Could you check a few things on this model? Use its own coordinates, in mm. Face numbers are marked on the shaded views. Coordinates: 2 decimals unless noted, no trailing zeros. Loops run counter-clockwise (first coordinate to the right, second up) from the corner with the lowest first, then second, coordinate; pieces in that order, holes last. Notation, with made-up numbers: (37.5, 73) - (62.5, 73) arc R10 cw to (62.5, 78) - close; hole circle Ø2 at (-3.5, 8.25). An arc over 180 degrees is marked (long way). Use CSV: the item, a comma, the result in double quotes.
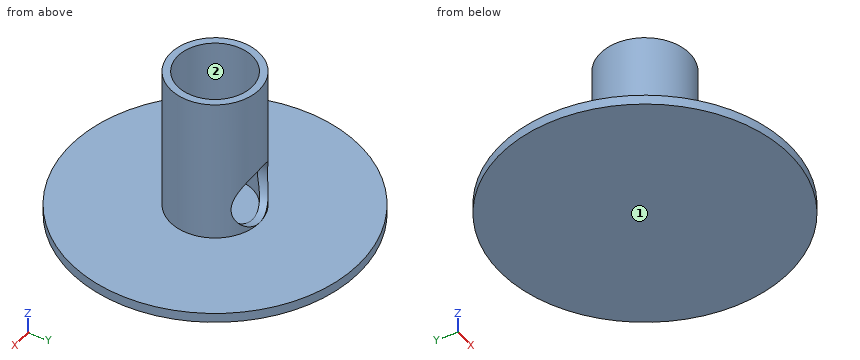
from build123d import *

# Parameters (mm, degrees)
F0_R     = 9.25
F0_R_2   = 7.75
F1_DEPTH = 30
F2_R     = 30
F3_DEPTH = 2
F4_R     = 6
F5_DEPTH = 25


with BuildPart() as f1:
    # F0 (on Top) → F1 (new body)
    with BuildSketch(Plane.XY):
        Circle(F0_R)
        Circle(F0_R_2, mode=Mode.SUBTRACT)
    extrude(amount=F1_DEPTH)

    # F2 (on face) → F3 (join)
    with BuildSketch(Plane(origin=(0, 0, 0), x_dir=(1, 0, 0), z_dir=(0, 0, -1))):
        Circle(F2_R)
    extrude(amount=F3_DEPTH)

    # F4 (on Front) → F5 (cut)
    with BuildSketch(Plane.XZ):
        with Locations((0, 6)):
            Circle(F4_R)
    extrude(amount=-F5_DEPTH, mode=Mode.SUBTRACT)


solid = f1.part
(1) Suppose I cut it at B-B (z = 25.5). Write out the boundary of the cut face in (x, y).
Computed:
outline,"circle Ø18.5 at (0, 0); hole circle Ø15.5 at (0, 0)"
(2) Thinking about a two-plate mould opening in X: for the marked faces 1 and 2, which applies, +X half, -X half, draft (parallel to the pull), parting line (faces both ways), or undercut?
Computed:
face 1,"draft"
face 2,"undercut"
(3) Suppose I cut it at A-A (y = 0). Write out the boundary of the cut face in (x, z).
Computed:
outline,"(-30, -2) - (30, -2) - (30, 0) - (9.25, 0) - (9.25, 30) - (7.75, 30) - (7.75, 0) - (-7.75, 0) - (-7.75, 30) - (-9.25, 30) - (-9.25, 0) - (-30, 0) - close"
(4) Please list where these lines run through material, in increasing order: line 1 (X direction, y = 0, z = 14); line 2 (Z direction, x = 5.5, y = 3.5).
Computed:
line 1,"x = -9.25 to -7.75, 7.75 to 9.25"
line 2,"z = -2 to 0"
(5) Suppose I cut it at C-C (z = 4.5). Write out the boundary of the cut face in (x, y), plus the area to 3 significant figures.
Computed:
outline,"(-5.81, 5.13) - (-5.81, 7.2) arc R9.25 ccw (long way) to (5.81, 7.2) - (5.81, 5.13) arc R7.75 cw (long way) to start"
area,"60.9 mm²"
(6) Will these pins go through, and if not, where does the flat tip stop? pin 1 (6 mm diameter, centred on y = 2.5, z = 8, fed in from -X); pin 2 (1.5 mm diameter, centred on y = -4, z = 11.5, fed in from -X); pin 3 (4 mm diameter, centred on x = 22, y = -1.5, fed in from +Z).
Computed:
pin 1,"stops at x = -9.25"
pin 2,"stops at x = -8.66"
pin 3,"stops at z = 0"
(7) Suppose I cut it at D-D (x = -14). Write out the boundary of the cut face in (y, z).
Computed:
outline,"(-26.53, -2) - (26.53, -2) - (26.53, 0) - (-26.53, 0) - close"
